Design review of the part shown in the three views and the two pictorial views. Dimensions are in mm from the part's minimum x, y and z. Coordinates: 2 decimals unless noted, no trailing zeros. Write each loop counter-clockwise with the first axis right and the second up, starting at its lowest first coordinate (ties: lowest second). Pieces come first, ordered by that corner, then holes. Notation, with made-up numbers: (56.25, 14) - (88.25, 14) arc R32 ccw to (88.25, 43) - close; hole circle Ø11 at (7.25, 78). An arc over 180 degrees is marked (long way). Return JSON: item names as keys, results as strings. Group by question number.
(1) We need section D-D on z = 11.5. State the section outline as (x, y) points.
(2) We need section A-A on y = 36.65. State the section outline as (x, z) points.
(3) To check wall thickness, follow L1, parallel to Y at x = 36.65, z = 7.75; L2, parallel to X at y = 4.5, z = 2.75; L3, parallel to X at y = 4, z = 2.5. State the ranges of each line that lie inside material, in increasing order. Write a range as from..to.
(4) For pin 1 Ø8 at (x, y) = (5.65, 5.65) entering from -Z; pin 2 Ø3 at (x, y) = (36.65, 5.65) entering from -Z, all flat-tipped, find the tip position at first contact; note any pin that passes through.
(5) We need section C-C on y = 21.15. State the section outline as (x, z) points.
(6) Draft analysis for pull direction X (two halves, no side actions). For the marked faces 1, 2, 3 and 4, state which applies: released by +X, released by -X, zero draft, split by the parting line, or undercut.
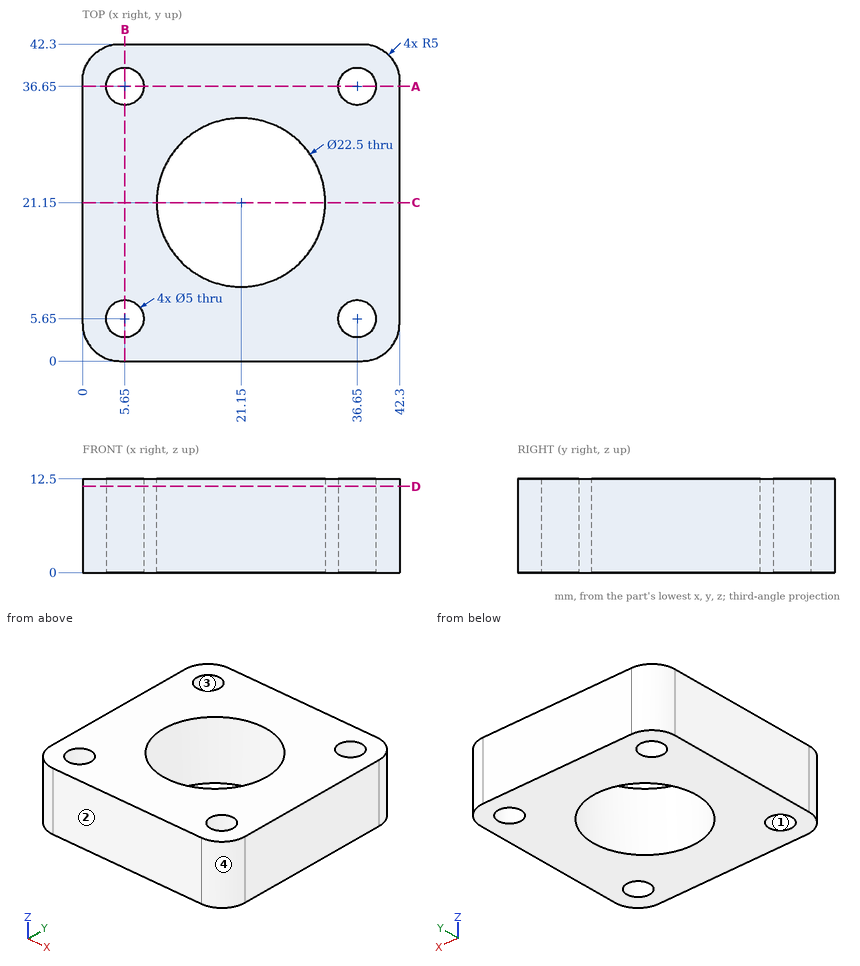
Ans:
{
 "1": {"outline": "(0, 5) arc R5 ccw to (5, 0) - (37.3, 0) arc R5 ccw to (42.3, 5) - (42.3, 37.3) arc R5 ccw to (37.3, 42.3) - (5, 42.3) arc R5 ccw to (0, 37.3) - close; hole circle Ø5 at (5.65, 5.65); hole circle Ø5 at (5.65, 36.65); hole circle Ø22.5 at (21.15, 21.15); hole circle Ø5 at (36.65, 5.65); hole circle Ø5 at (36.65, 36.65)"},
 "2": {"outline": "(0, 0) - (3.15, 0) - (3.15, 12.5) - (0, 12.5) - close; (8.15, 0) - (34.15, 0) - (34.15, 12.5) - (8.15, 12.5) - close; (39.15, 0) - (42.3, 0) - (42.3, 12.5) - (39.15, 12.5) - close"},
 "3": {"L1": "0..3.15, 8.15..34.15, 39.15..42.3", "L2": "0.03..3.43, 7.87..34.43, 38.87..42.27", "L3": "0.1..3.77, 7.53..34.77, 38.53..42.2"},
 "4": {"pin 1": "z = 0", "pin 2": "through"},
 "5": {"outline": "(0, 0) - (9.9, 0) - (9.9, 12.5) - (0, 12.5) - close; (32.4, 0) - (42.3, 0) - (42.3, 12.5) - (32.4, 12.5) - close"},
 "6": {"face 1": "undercut", "face 2": "zero draft", "face 3": "undercut", "face 4": "released by +X"}
}
